from build123d import *

# Parameters (mm, degrees)
SKETCH1_W           = 25
SKETCH1_H           = 15
BOSS_EXTRUDE1_DEPTH = 15
SKETCH2_W           = 20
SKETCH2_H           = 13
CUT_EXTRUDE1_DEPTH  = 13
SKETCH3_W           = 19
SKETCH3_H           = 12
CUT_EXTRUDE2_DEPTH  = 33.787192622
SKETCH10_W          = 11
SKETCH10_H          = 3
BOSS_EXTRUDE5_DEPTH = 10
SKETCH11_R          = 1.5
CUT_EXTRUDE4_DEPTH  = 32.527765541
SKETCH13_W          = 11
SKETCH13_H          = 3
BOSS_EXTRUDE6_DEPTH = 10
SKETCH14_R          = 1.5
CUT_EXTRUDE5_DEPTH  = 40.924929555


with BuildPart() as part:
    # Sketch1 → Boss-Extrude1 (new body)
    with BuildSketch(Plane.XY):
        with Locations((12.5, -7.5)):
            Rectangle(SKETCH1_W, SKETCH1_H)
    extrude(amount=BOSS_EXTRUDE1_DEPTH)

    # Sketch2 → Cut-Extrude1 (cut)
    with BuildSketch(Plane(origin=(0, 0, 0), x_dir=(-1, 0, 0), z_dir=(0, 0, -1))):
        with Locations((-12.5, -7.5)):
            Rectangle(SKETCH2_W, SKETCH2_H)
    extrude(amount=-CUT_EXTRUDE1_DEPTH, mode=Mode.SUBTRACT)

    # Sketch3 → Cut-Extrude2 (cut, through all)
    with BuildSketch(Plane.XY.offset(15)):
        with Locations((12.5, -7.5)):
            Rectangle(SKETCH3_W, SKETCH3_H)
    extrude(amount=-CUT_EXTRUDE2_DEPTH, mode=Mode.SUBTRACT)

    # Sketch10 → Boss-Extrude5 (add)
    with BuildSketch(Plane.ZY):
        with Locations((7.5, -13.5)):
            Rectangle(SKETCH10_W, SKETCH10_H)
    extrude(amount=BOSS_EXTRUDE5_DEPTH)

    # Sketch11 → Cut-Extrude4 (cut, through all)
    with BuildSketch(Plane(origin=(0, -12, 0), x_dir=(1, 0, 0), z_dir=(0, 1, 0))):
        with Locations(Location((-5, -7.5, 0), (0, 0, 180))):
            Circle(SKETCH11_R)
    extrude(amount=-CUT_EXTRUDE4_DEPTH, mode=Mode.SUBTRACT)

    # Sketch13 → Boss-Extrude6 (add)
    with BuildSketch(Plane(origin=(25, 0, 0), x_dir=(0, 0, -1), z_dir=(1, 0, 0))):
        with Locations((-7.5, -13.5)):
            Rectangle(SKETCH13_W, SKETCH13_H)
    extrude(amount=BOSS_EXTRUDE6_DEPTH)

    # Sketch14 → Cut-Extrude5 (cut, through all)
    with BuildSketch(Plane(origin=(0, -12, 0), x_dir=(1, 0, 0), z_dir=(0, 1, 0))):
        with Locations(Location((30, -7.5, 0), (0, 0, 180))):
            Circle(SKETCH14_R)
    extrude(amount=-CUT_EXTRUDE5_DEPTH, mode=Mode.SUBTRACT)


solid = part.part
The model under review builds one solid part; all positions refer to its coordinate system, in mm. A direction names the side the tool comes from. Coordinates: 2 decimals unless noted, no trailing zeros. Loops run counter-clockwise (first coordinate to the right, second up) from the corner with the lowest first, then second, coordinate; pieces in that order, holes last. Notation, with made-up numbers: M 63.25,68 L 89.25,68 A24 cw 89.25,103 Z; hole C 16.25,74 d9. An arc over 180 degrees is marked long. Put each result on its own line as item: value. Start each with the question number.
Q1. Clearance check with flat-ended pins moving along their axes: pin 1 (0.6 mm diameter, centred on y = -8, z = 14, fed in from +X); pin 2 (1 mm diameter, centred on x = 29.5, z = 6, fed in from +Y); pin 3 (3.5 mm diameter, centred on x = -5.5, y = -13, fed in from +Z). State where each tip first meets the part, or that it passes through.
Q2. Add section C-C (x = 30). Write out the cut boundary in (y, z), and give its area (3 significant figures).
Q3. Wall thickness on line 1 (Z direction, x = 30, y = -12.9); line 2 (X direction, y = -8.25, z = 9.25); line 3 (Y direction, x = 7, z = 11): over which ranges is each line inside the solid? List them lowest first.
Q4. Add section B-B (y = -12.5). Write out the cut boundary in (x, z).
Q5. Add section D-D (z = 4). Write out the cut boundary in (x, y), and give its area (3 significant figures).
Q6. The part is to be moulded in two halves that separate along Y. For faces 5 (the flat face through (12, -13.5, 14)), 6 (the flat face through (-10, -13, 7)), 7 (the flat face through (-4, -12, 9)), 8 (the flat face through (3, -8, 14)), say which applies: +Y half, -Y half, draft (parallel to the pull), parting line (faces both ways), or undercut.
Q7. Add section A-A (z = 7.5). Write out the cut boundary in (x, y).
Q8. For faces 1 (the flat face through (-5, -14, 2)), 2 (the flat face through (22, -8, 14)), 3 (the flat face through (30, -14, 2)), 4 (the flat face through (30, -14, 13)), list the 3-axis set-ups (+Z, -Z, +X, -X, +Y, -Y) from which the entire face can be reached by the end or side of a thin tool; tool diameter is ignored.
Answers:
1. pin 1: stops at x = 25
1. pin 2: stops at y = -12
1. pin 3: stops at z = 13
2. outline: M -15,2 L -12,2 L -12,6 L -15,6 Z; M -15,9 L -12,9 L -12,13 L -15,13 Z
2. area: 24.0 mm^2
3. line 1: z = 2 to 6, 9 to 13
3. line 2: x = 0 to 2.5, 22.5 to 25
3. line 3: y = -15 to -14, -1 to 0
4. outline: M -10,2 L 0,2 L 0,0 L 2.5,0 L 2.5,13 L 3,13 L 3,15 L 0,15 L 0,13 L -10,13 Z; M 22,13 L 22.5,13 L 22.5,0 L 25,0 L 25,2 L 35,2 L 35,13 L 25,13 L 25,15 L 22,15 Z; hole C -5,7.5 d3; hole C 30,7.5 d3
5. outline: M -10,-15 L 35,-15 L 35,-12 L 25,-12 L 25,0 L 0,0 L 0,-12 L -10,-12 Z; hole M 2.5,-14 L 22.5,-14 L 22.5,-1 L 2.5,-1 Z
5. area: 175 mm^2
6. face 5: undercut
6. face 6: draft
6. face 7: +Y half
6. face 8: undercut
7. outline: M -10,-15 L -6.5,-15 L -6.5,-12 L -10,-12 Z; M -3.5,-15 L 28.5,-15 L 28.5,-12 L 25,-12 L 25,0 L 0,0 L 0,-12 L -3.5,-12 Z; M 31.5,-15 L 35,-15 L 35,-12 L 31.5,-12 Z; hole M 2.5,-14 L 22.5,-14 L 22.5,-1 L 2.5,-1 Z
8. face 1: -Z, -X, +Y, -Y
8. face 2: +Z, -Z
8. face 3: -Z, +X, +Y, -Y
8. face 4: +Z, +X, +Y, -Y
